Could you check a few things on this model? Use its own coordinates, in mm. Face numbers are marked on the shaded views. A direction names the side the tool comes from. Round coordinates to 2 decimals unless told otherwise and drop trailing zeros. Write each loop counter-clockwise with the first axis right and the second up, starting at its lowest first coordinate (ties: lowest second). Pieces come first, ordered by that corner, then holes. Notation, with made-up numbers: (68, 26.5) -> (110, 26.5) arc R33 cw to (110, 64.5) -> close; hole circle Ø8 at (63.25, 3). An arc over 180 degrees is marked (long way). Answer in a Markdown table with one row per item.
from build123d import *

# Parameters (mm, degrees)
F0_W      = 50.8
F0_H      = 50.8
F1_DEPTH  = 12.7
F5_D      = 6.35
F5_DEPTH  = 20.6375
F5_TIP    = 1.9077324654
F7_D      = 3.7973
F8_R      = 1.190625
F9_DEPTH  = 3.81
F10_R     = 1.190625
F11_DEPTH = 12.701


with BuildPart() as f1:
    # F0 (on Top) → F1 (new body)
    with BuildSketch(Plane.XY):
        Rectangle(F0_W, F0_H)
    extrude(amount=F1_DEPTH)

    # F5
    with Locations(Plane(origin=(-25.4, 0, 0), x_dir=(0, -1, 0), z_dir=(-1, 0, 0))):
        with Locations((0, 4.445)):
            Hole(F5_D / 2, depth=F5_DEPTH)
            with Locations((0, 0, -(F5_DEPTH + F5_TIP / 2))):  # 118° drill point
                Cone(0, F5_D / 2, F5_TIP, mode=Mode.SUBTRACT)

    # F7 (through all)
    with Locations(Plane.XY.offset(12.7)):
        with Locations((-19.05, 19.05), (19.05, 19.05), (19.05, -19.05), (-19.05, -19.05)):
            Hole(F7_D / 2)

    # F8 (on face) → F9 (cut)
    with BuildSketch(Plane.XY.offset(12.7)):
        with BuildLine():
            Line((20.6375, 8.5292954232), (20.6375, 10.80135))
            ThreePointArc((20.6375, 10.80135), (20.1725320151, 11.9238820151), (19.05, 12.38885))
            ThreePointArc((19.05, 12.38885), (14.3398556645, 14.3398556645), (12.38885, 19.05))
            ThreePointArc((12.38885, 19.05), (11.9238820151, 20.1725320151), (10.80135, 20.6375))
            Line((10.80135, 20.6375), (-10.80135, 20.6375))
            ThreePointArc((-10.80135, 20.6375), (-11.9238820151, 20.1725320151), (-12.38885, 19.05))
            ThreePointArc((-12.38885, 19.05), (-14.3398556645, 14.3398556645), (-19.05, 12.38885))
            ThreePointArc((-19.05, 12.38885), (-20.1725320151, 11.9238820151), (-20.6375, 10.80135))
            Line((-20.6375, 10.80135), (-20.6375, -10.80135))
            ThreePointArc((-20.6375, -10.80135), (-20.1725320151, -11.9238820151), (-19.05, -12.38885))
            ThreePointArc((-19.05, -12.38885), (-14.3398556645, -14.3398556645), (-12.38885, -19.05))
            ThreePointArc((-12.38885, -19.05), (-11.9238820151, -20.1725320151), (-10.80135, -20.6375))
            Line((-10.80135, -20.6375), (10.80135, -20.6375))
            ThreePointArc((10.80135, -20.6375), (11.9238820151, -20.1725320151), (12.38885, -19.05))
            ThreePointArc((12.38885, -19.05), (14.3398556645, -14.3398556645), (19.05, -12.38885))
            ThreePointArc((19.05, -12.38885), (20.1725320151, -11.9238820151), (20.6375, -10.80135))
            Line((20.6375, -10.80135), (20.6375, 4.5605454232))
            ThreePointArc((20.6375, 4.5605454232), (20.1725320151, 5.6830774384), (19.05, 6.1480454232))
            Line((19.05, 6.1480454232), (14.2875, 6.1480454232))
            Line((14.2875, 6.1480454232), (14.2875, 6.0926137759))
            ThreePointArc((14.2875, 6.0926137759), (9.9452262, 8.6731816985), (6.821921312, 12.643022896))
            ThreePointArc((6.821921312, 12.643022896), (6.2374933843, 13.2645178717), (5.4157485098, 13.49375))
            Line((5.4157485098, 13.49375), (-5.4157485098, 13.49375))
            ThreePointArc((-5.4157485098, 13.49375), (-6.2374933843, 13.2645178717), (-6.821921312, 12.643022896))
            ThreePointArc((-6.821921312, 12.643022896), (-9.2884615964, 9.2884615964), (-12.643022896, 6.821921312))
            ThreePointArc((-12.643022896, 6.821921312), (-13.2645178717, 6.2374933843), (-13.49375, 5.4157485098))
            Line((-13.49375, 5.4157485098), (-13.49375, -5.4157485098))
            ThreePointArc((-13.49375, -5.4157485098), (-13.2645178717, -6.2374933843), (-12.643022896, -6.821921312))
            ThreePointArc((-12.643022896, -6.821921312), (-9.2884615964, -9.2884615964), (-6.821921312, -12.643022896))
            ThreePointArc((-6.821921312, -12.643022896), (-6.2374933843, -13.2645178717), (-5.4157485098, -13.49375))
            Line((-5.4157485098, -13.49375), (5.4157485098, -13.49375))
            ThreePointArc((5.4157485098, -13.49375), (6.2374933843, -13.2645178717), (6.821921312, -12.643022896))
            ThreePointArc((6.821921312, -12.643022896), (9.2884615964, -9.2884615964), (12.643022896, -6.821921312))
            ThreePointArc((12.643022896, -6.821921312), (13.2645178717, -6.2374933843), (13.49375, -5.4157485098))
            Line((13.49375, -5.4157485098), (13.49375, -2.3239302132))
            ThreePointArc((13.49375, -2.3239302132), (13.1944701574, -1.3962206272), (12.4094727388, -0.8182997389))
            ThreePointArc((12.4094727388, -0.8182997389), (7.1639891354, 1.7998207966), (2.8493973076, 5.7689454776))
            ThreePointArc((2.8493973076, 5.7689454776), (2.3008328233, 6.1974021649), (1.6217068945, 6.35))
            Line((1.6217068945, 6.35), (-1.6217068945, 6.35))
            ThreePointArc((-1.6217068945, 6.35), (-2.3008328233, 6.1974021649), (-2.8493973076, 5.7689454776))
            ThreePointArc((-2.8493973076, 5.7689454776), (-4.2370675283, 4.2370675283), (-5.7689454776, 2.8493973076))
            ThreePointArc((-5.7689454776, 2.8493973076), (-6.1974021649, 2.3008328233), (-6.35, 1.6217068945))
            Line((-6.35, 1.6217068945), (-6.35, -1.6217068945))
            ThreePointArc((-6.35, -1.6217068945), (-6.1974021649, -2.3008328233), (-5.7689454776, -2.8493973076))
            ThreePointArc((-5.7689454776, -2.8493973076), (-4.2370675283, -4.2370675283), (-2.8493973076, -5.7689454776))
            ThreePointArc((-2.8493973076, -5.7689454776), (-2.3008328233, -6.1974021649), (-1.6217068945, -6.35))
            Line((-1.6217068945, -6.35), (1.6217068945, -6.35))
            ThreePointArc((1.6217068945, -6.35), (2.3008328233, -6.1974021649), (2.8493973076, -5.7689454776))
            ThreePointArc((2.8493973076, -5.7689454776), (3.6282714753, -4.8719808812), (4.4567370697, -4.0206083333))
            ThreePointArc((4.4567370697, -4.0206083333), (4.8051043626, -4.2373192983), (5.1566891771, -4.4487703125))
            ThreePointArc((5.1566891771, -4.4487703125), (3.9121206801, -5.7434375699), (2.7877367827, -7.14375))
            Line((2.7877367827, -7.14375), (-2.7877367827, -7.14375))
            ThreePointArc((-2.7877367827, -7.14375), (-4.7983335359, -4.7983335359), (-7.14375, -2.7877367827))
            Line((-7.14375, -2.7877367827), (-7.14375, 2.7877367827))
            ThreePointArc((-7.14375, 2.7877367827), (-4.7983335359, 4.7983335359), (-2.7877367827, 7.14375))
            Line((-2.7877367827, 7.14375), (2.7877367827, 7.14375))
            ThreePointArc((2.7877367827, 7.14375), (7.858589431, 2.2877709273), (14.2875, -0.5341412311))
            Line((14.2875, -0.5341412311), (14.2875, -6.9417954232))
            ThreePointArc((14.2875, -6.9417954232), (9.849727604, -9.849727604), (6.9417954232, -14.2875))
            Line((6.9417954232, -14.2875), (-6.9417954232, -14.2875))
            ThreePointArc((-6.9417954232, -14.2875), (-9.849727604, -9.849727604), (-14.2875, -6.9417954232))
            Line((-14.2875, -6.9417954232), (-14.2875, 6.9417954232))
            ThreePointArc((-14.2875, 6.9417954232), (-9.849727604, 9.849727604), (-6.9417954232, 14.2875))
            Line((-6.9417954232, 14.2875), (6.9417954232, 14.2875))
            ThreePointArc((6.9417954232, 14.2875), (9.849727604, 9.849727604), (14.2875, 6.9417954232))
            Line((14.2875, 6.9417954232), (19.05, 6.9417954232))
            ThreePointArc((19.05, 6.9417954232), (20.1725320151, 7.4067634081), (20.6375, 8.5292954232))
        make_face()
        with Locations((-1.778, -4.7625)):
            Circle(F8_R, mode=Mode.SUBTRACT)
        with Locations((1.778, -4.7625)):
            Circle(F8_R, mode=Mode.SUBTRACT)
        with Locations((-1.778, 4.7625)):
            Circle(F8_R, mode=Mode.SUBTRACT)
        with Locations((1.778, 4.7625)):
            Circle(F8_R, mode=Mode.SUBTRACT)
        with Locations((-1.778, 4.7625)):
            Circle(F8_R)
        with Locations((1.778, 4.7625)):
            Circle(F8_R)
        with Locations((1.778, -4.7625)):
            Circle(F8_R)
        with Locations((-1.778, -4.7625)):
            Circle(F8_R)
    extrude(amount=-F9_DEPTH, mode=Mode.SUBTRACT)

    # F10 (on face) → F11 (cut, through all)
    with BuildSketch(Plane.XY.offset(12.7)):
        with Locations((-1.778, 4.7625)):
            Circle(F10_R)
        with Locations((1.778, 4.7625)):
            Circle(F10_R)
        with Locations((1.778, -4.7625)):
            Circle(F10_R)
        with Locations((-1.778, -4.7625)):
            Circle(F10_R)
    extrude(amount=-F11_DEPTH, mode=Mode.SUBTRACT)


solid = f1.part
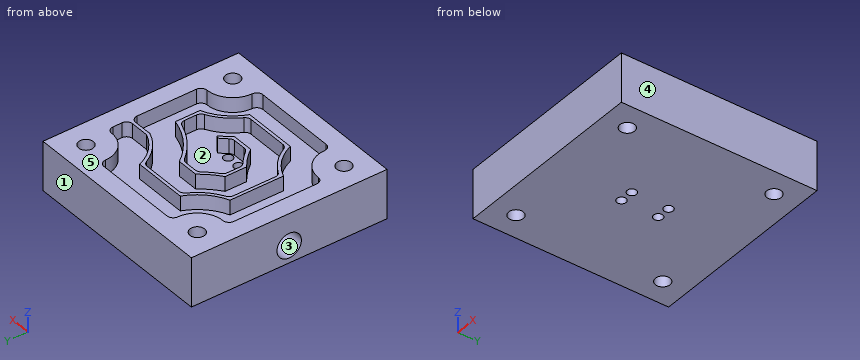
1) Imagine slicing it at B-B, the plane z = 10. Count the separate pieces of the cut face and the enclosed holes in it, plus the area to 3 significant figures.
Findings:
| item | result |
|---|---|
| separate pieces | 1 |
| enclosed holes | 5 |
| area | 1,180 mm^2 |
2) For pin 1 (2 mm diameter, centred on x = -0.5, y = 2, fed in from +Z); pin 2 (3.5 mm diameter, centred on x = -19.05, y = -19.05, fed in from -Z), each with a flat end and sliding along its axis, tell me the tip position at first contact or that it passes through.
Findings:
| item | result |
|---|---|
| pin 1 | stops at z = 8.89 |
| pin 2 | passes through |
3) For the marked faces 1 and 2, which set-ups out of +Z, -Z, +X, -X, +Y, -Y let a thin tool reach every point of the face, with its end or its side?
Findings:
| item | result |
|---|---|
| face 1 | +Z, -Z, +X, -X, +Y |
| face 2 | +Z |
4) Imagine slicing it at C-C, the plane y = 15.5. Please give me the cut outline in (x, z).
Findings:
| item | result |
|---|---|
| outline | (-25.4, 0) -> (25.4, 0) -> (25.4, 12.7) -> (13.41, 12.7) -> (13.41, 8.89) -> (-13.41, 8.89) -> (-13.41, 12.7) -> (-25.4, 12.7) -> close |
5) Imagine slicing it at A-A, the plane x = 0. Please give me the cut outline in (y, z), plus the area to 3 significant figures.
Findings:
| item | result |
|---|---|
| outline | (-25.4, 0) -> (25.4, 0) -> (25.4, 12.7) -> (20.64, 12.7) -> (20.64, 8.89) -> (14.29, 8.89) -> (14.29, 12.7) -> (13.49, 12.7) -> (13.49, 8.89) -> (7.14, 8.89) -> (7.14, 12.7) -> (6.35, 12.7) -> (6.35, 8.89) -> (-6.35, 8.89) -> (-6.35, 12.7) -> (-7.14, 12.7) -> (-7.14, 8.89) -> (-13.49, 8.89) -> (-13.49, 12.7) -> (-14.29, 12.7) -> (-14.29, 8.89) -> (-20.64, 8.89) -> (-20.64, 12.7) -> (-25.4, 12.7) -> close |
| area | 500 mm^2 |
6) Please list where these lines run through material, in increasing order: line 1 (Y direction, x = 19.05, z = 7.75); line 2 (X direction, y = 8.5, z = 11.25); line 3 (Y direction, x = 16, z = 9.5).
Findings:
| item | result |
|---|---|
| line 1 | y = -25.4 to -20.95, -17.15 to 17.15, 20.95 to 25.4 |
| line 2 | x = -25.4 to -20.64, -11.44 to -10.15, 10.15 to 11.44, 20.64 to 25.4 |
| line 3 | y = -25.4 to -13.13, 6.15 to 6.94, 13.13 to 25.4 |
7) Thinking about a two-plate mould opening in Z: for the marked faces 3, 4 and 5, which applies, +Z half, -Z half, draft (parallel to the pull), parting line (faces both ways), or undercut?
Findings:
| item | result |
|---|---|
| face 3 | undercut |
| face 4 | draft |
| face 5 | +Z half |
